Verification items for this drawing (mm, ordinates from the low corner). A direction names the side the tool comes from. Coordinates: 2 decimals unless noted, no trailing zeros. Order: outer loops, then holes, each group sorted by start corner. A loop starts at its lowest first (then second) coordinate and runs counter-clockwise, first axis right, second up. Notation, with made-up numbers: (-23, 78) - (-13, 78) arc R25 cw to (-13, 102) - close; hole circle Ø10 at (72, 44.5). An arc over 180 degrees is marked (long way). One line per question, with ' | ' between items. Start each with the question number.
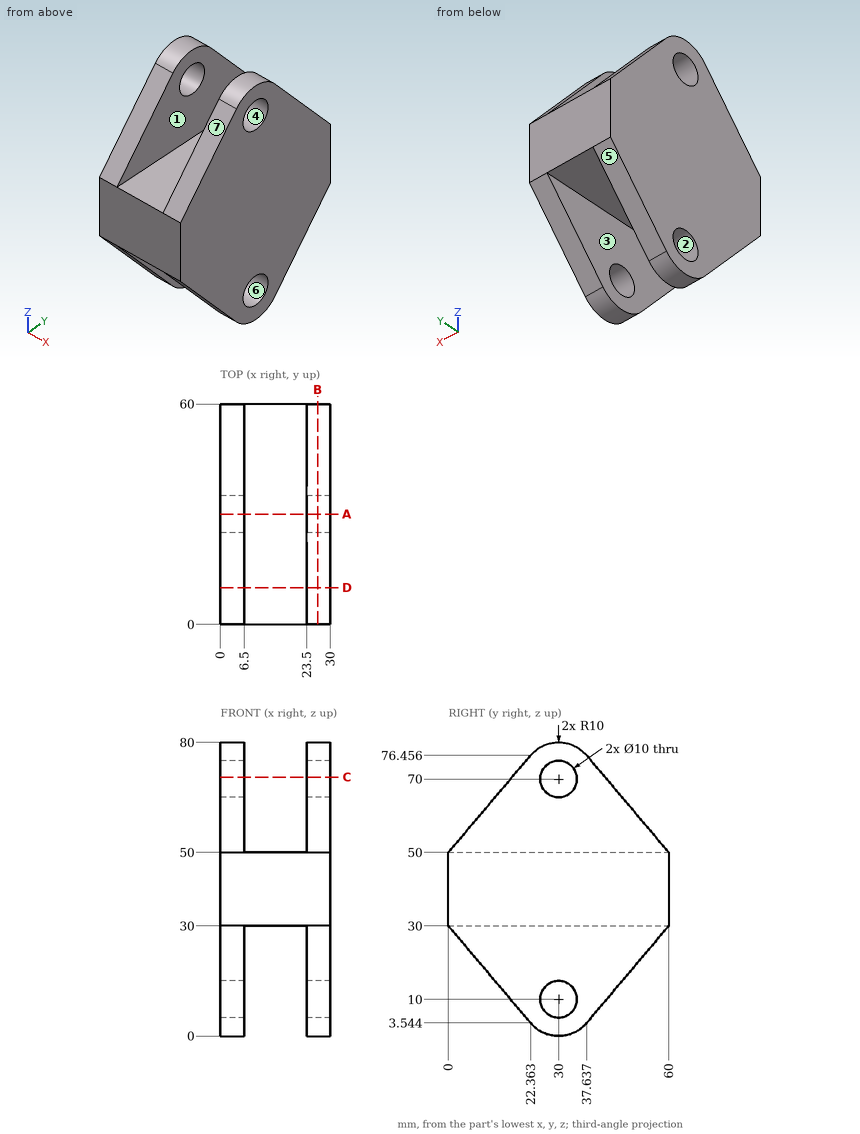
Item 1: Section check A-A (y = 30). Record the cut outline in (x, z).
Item 2: Set-up check for the marked faces 1, 2 and 3: record each of +Z, -Z, +X, -X, +Y, -Y from which the full face is reachable in a straight line by a thin tool's end or side.
Item 3: Gauge pin test, flat ends, axial feed: pin 1 (9 mm diameter, centred on y = 26, z = 21.5, fed in from -X); pin 2 (8 mm diameter, centred on x = 7.5, z = 67.5, fed in from -Y); pin 3 (6 mm diameter, centred on x = 5, y = 8.5, fed in from -Z) (1 decimal); pin 4 (5 mm diameter, centred on x = 12, y = 26.5, fed in from +Z). Record the tip position at first contact, or that the pin passes through.
Item 4: Section check C-C (z = 70.5). Record the cut outline in (x, y) (1 decimal).
Item 5: Mould release check, pull along Z, two halves, no side actions. Record for the marked faces 4, 5, 6 and 7: +Z half, -Z half, draft (parallel to the pull), parting line (faces both ways), or undercut.
Item 6: Section check D-D (y = 10). Record the cut outline in (x, z).
Item 7: Thickness scan on probe 1 along X at (y, z) = (50.5, 24.5); probe 2 along Z at (x, y) = (15, 54); probe 3 along Y at (x, z) = (5.25, 74.5). Record the ranges inside material, lowest first. Write a range as from..to.
Item 8: Section check B-B (x = 26.5). Record the cut outline in (y, z) (1 decimal), then the cut area to 3 significant figures.
Completed:
1) outline: (0, 0) - (6.5, 0) - (6.5, 5) - (0, 5) - close; (0, 15) - (6.5, 15) - (6.5, 30) - (23.5, 30) - (23.5, 15) - (30, 15) - (30, 65) - (23.5, 65) - (23.5, 50) - (6.5, 50) - (6.5, 65) - (0, 65) - close; (0, 75) - (6.5, 75) - (6.5, 80) - (0, 80) - close; (23.5, 0) - (30, 0) - (30, 5) - (23.5, 5) - close; (23.5, 75) - (30, 75) - (30, 80) - (23.5, 80) - close
2) face 1: +Z, +Y, -Y | face 2: +X, -X | face 3: -Z, +Y, -Y
3) pin 1: stops at x = 0 | pin 2: stops at y = 11.52 | pin 3: stops at z = 16.4 | pin 4: stops at z = 50
4) outline: (0, 17.3) - (6.5, 17.3) - (6.5, 25) - (0, 25) - close; (0, 35) - (6.5, 35) - (6.5, 42.7) - (0, 42.7) - close; (23.5, 17.3) - (30, 17.3) - (30, 25) - (23.5, 25) - close; (23.5, 35) - (30, 35) - (30, 42.7) - (23.5, 42.7) - close
5) face 4: undercut | face 5: -Z half | face 6: undercut | face 7: +Z half
6) outline: (0, 18.17) - (6.5, 18.17) - (6.5, 30) - (23.5, 30) - (23.5, 18.17) - (30, 18.17) - (30, 61.83) - (23.5, 61.83) - (23.5, 50) - (6.5, 50) - (6.5, 61.83) - (0, 61.83) - close
7) probe 1: x = 0..6.5, 23.5..30 | probe 2: z = 30..50 | probe 3: y = 20.71..27.82, 32.18..39.29
8) outline: (0, 30) - (22.4, 3.5) arc R10 ccw to (37.6, 3.5) - (60, 30) - (60, 50) - (37.6, 76.5) arc R10 ccw to (22.4, 76.5) - (0, 50) - close; hole circle Ø10 at (30, 10); hole circle Ø10 at (30, 70) | area: 3,110 mm^2
